Autodesk Inventor part; units mm, degrees
ref_plane "YZ Plane" through (0, 0, 0) normal (1, 0, 0) x (0, 1, 0)
ref_plane "XZ Plane" through (0, 0, 0) normal (0, 1, 0) x (-1, 0, 0)
ref_plane "XY Plane" through (0, 0, 0) normal (0, 0, 1) x (1, 0, 0)
sketch "Sketch1" plane through (0, 0, 0) normal (0, 0, 1) x (1, 0, 0)
  circle A0 centre (0, 0) radius 14.65
  dimension "d0" = 29.3
extrude "Extrusion1" add sketch "Sketch1" along normal blind 5.5
chamfer "Chamfer1" distance 0.5 angle 45 2 edges at (-14.65, 0, 5.5) (-14.65, 0, 0)
sketch "Sketch2" plane through (0, 0, 5.5) normal (0, 0, 1) x (1, 0, 0)
  circle A0 centre (0, 0) radius 14.65
hole "Hole1" at (0, 0, 5.5) direction (0, 0, -1) diameter 8.5 depth 8 tip angle 118 countersink diameter 17.3 countersink angle 90
properties part number "ring wiel" material "Stainless Steel"
The listing builds one solid part. Answer for the finished solid, in the listing's coordinates (mm). Coordinates: 2 decimals unless noted, no trailing zeros. Loops run counter-clockwise (first coordinate to the right, second up) from the corner with the lowest first, then second, coordinate; pieces in that order, holes last. Notation, with made-up numbers: (87, 8.25) -> (144, 8.25) arc R34 ccw to (144, 44.25) -> close; hole circle Ø2 at (53.25, -6.5). An arc over 180 degrees is marked (long way). Answer in a Markdown table with one row per item. Add a question column.
1. The part is cut by section C-C, the plane z = 2.1. Write down the section's boundary in (x, y).
2. Consider line 1 (Y direction, x = 0, z = 0.5); line 2 (X direction, y = 3.25, z = 4.5); line 3 (Y direction, x = 2.75, z = 1.2). Determine where each line is inside the solid, lowest interval first. Write a range as [from, to].
3. Determine the mould class of faces 1 (the flat face through (-6.5, -6.1, 5.5)), 2 (the conical face through (-4.42, 0.98, 1.38)), 3 (the cylindrical face through (13.973, -4.4, 2.718)), 4 (the cylindrical face through (-3.584, -2.285, 0.542)) for opening direction X: +X half, -X half, draft (parallel to the pull), parting line (faces both ways), or undercut.
4. Flat-ended cylindrical pins translate along their axes: P1, Ø1, axis at x = -11, z = 2.5, coming from the +Y side; P2, Ø3, axis at x = 11.5, z = 3, coming from the +Y side; P3, Ø3, axis at x = 9.5, z = 5, coming from the -Y side. Find the tip coordinate at first contact, or state that the pin passes through.
5. The part is cut by section A-A, the plane x = 0. Write down the section's boundary in (y, z).
Answer below:
| question | item | result |
|---|---|---|
| 1 | outline | circle Ø29.3 at (0, 0); hole circle Ø10.5 at (0, 0) |
| 2 | line 1 | [-14.65, -4.25], [4.25, 14.65] |
| 2 | line 2 | [-14.28, -6.93], [6.93, 14.28] |
| 2 | line 3 | [-14.39, -3.37], [3.37, 14.39] |
| 3 | face 1 | draft |
| 3 | face 2 | undercut |
| 3 | face 3 | parting line |
| 3 | face 4 | undercut |
| 4 | P1 | y = 10.22 |
| 4 | P2 | y = 10.71 |
| 4 | P3 | y = -12.27 |
| 5 | outline | (-14.65, 0.5) -> (-14.15, 0) -> (-4.25, 0) -> (-4.25, 1.1) -> (-8.65, 5.5) -> (-14.15, 5.5) -> (-14.65, 5) -> close; (4.25, 0) -> (14.15, 0) -> (14.65, 0.5) -> (14.65, 5) -> (14.15, 5.5) -> (8.65, 5.5) -> (4.25, 1.1) -> close |
